Check sheet for the drawn part. Datum: minimum x, y, z corner. Units: mm. A direction names the side the tool comes from. Coordinates: 2 decimals unless noted, no trailing zeros. Write each loop counter-clockwise with the first axis right and the second up, starting at its lowest first coordinate (ties: lowest second). Pieces come first, ordered by that corner, then holes. Notation, with made-up numbers: (-13.5, 68.25) -> (-4.5, 68.25) arc R10 cw to (-4.5, 81.25) -> close; hole circle Ø2 at (70, 52). An arc over 180 degrees is marked (long way). Answer in a Markdown table with one row per item. Add a question column.
Q1. Gauge pin test, flat end, axial feed: P1, Ø8, axis at x = 259, y = 422, coming from the +Z side. Record the tip position at first contact, or that the pin passes through.
Q2. Section check A-A, the plane z = 137. Record the boundary of the cut face in (x, y).
Q3. Section check C-C, the plane y = 432.5. Record the boundary of the cut face in (x, z).
Q4. Section check B-B, the plane x = 274. Record the boundary of the cut face in (y, z).
Q5. Thickness scan on line 1 (Y direction, x = 122, z = 104); line 2 (X direction, y = 297.5, z = 88.5); line 3 (Z direction, x = 288, y = 260). Record the ranges inside material, lowest first.
Q6. Tool access check on the marked faces 5 and 6. Record the directions out of +Z, -Z, +X, -X, +Y, -Y that give a thin tool (end or side, any length) a straight path to the whole face; none if there is none.
Q7. Release check for a two-part mould opening along Y. For the marked faces 1, 2, 3 and 4 record: pulls with the +Y half, pulls with the -Y half, needs draft (parallel to the pull), parting line crosses it, or undercut.
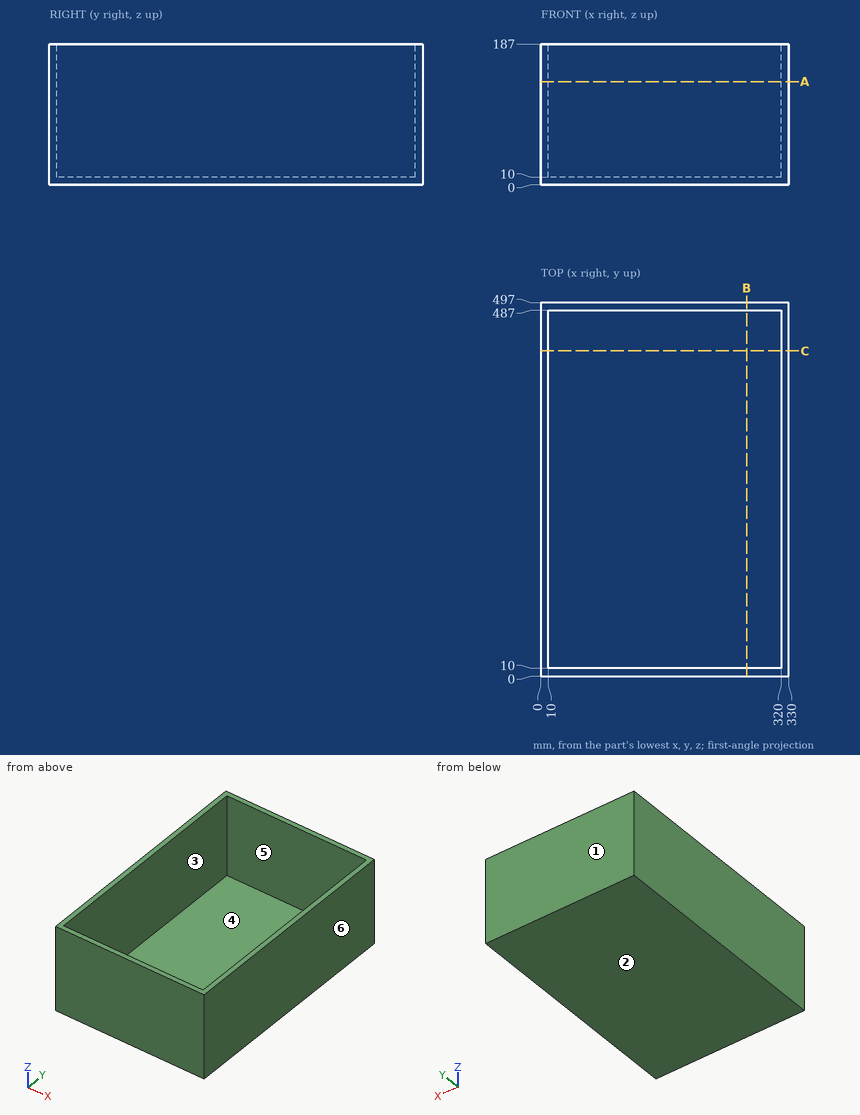
Calculated:
| question | item | result |
|---|---|---|
| 1 | P1 | stops at z = 10 |
| 2 | outline | (0, 0) -> (330, 0) -> (330, 497) -> (0, 497) -> close; hole (10, 10) -> (320, 10) -> (320, 487) -> (10, 487) -> close |
| 3 | outline | (0, 0) -> (330, 0) -> (330, 187) -> (320, 187) -> (320, 10) -> (10, 10) -> (10, 187) -> (0, 187) -> close |
| 4 | outline | (0, 0) -> (497, 0) -> (497, 187) -> (487, 187) -> (487, 10) -> (10, 10) -> (10, 187) -> (0, 187) -> close |
| 5 | line 1 | y = 0 to 10, 487 to 497 |
| 5 | line 2 | x = 0 to 10, 320 to 330 |
| 5 | line 3 | z = 0 to 10 |
| 6 | face 5 | +Z |
| 6 | face 6 | +Z, -Z, +X, +Y, -Y |
| 7 | face 1 | pulls with the +Y half |
| 7 | face 2 | needs draft |
| 7 | face 3 | undercut |
| 7 | face 4 | undercut |
